The model under review builds one solid part; all positions refer to its coordinate system, in mm. Round coordinates to 2 decimals unless told otherwise and drop trailing zeros. Order: outer loops, then holes, each group sorted by start corner. A loop starts at its lowest first (then second) coordinate and runs counter-clockwise, first axis right, second up. Notation, with made-up numbers: (4, 83) - (35, 83) arc R12 ccw to (35, 91) - close; hole circle Ø11 at (-22, 4). An arc over 180 degrees is marked (long way). One line per question, with ' | ' between items. Start each with the question number.
Item 1: Add section B-B on z = 6. State the section outline as (x, y) points.
Item 2: For L1, parallel to X at y = -23, z = 7.75; L2, parallel to Y at x = -41, z = 1; L3, parallel to Y at x = 123.5, z = 4.75, list the stretches that pass through material, from the lowest coordinate up. Write a range as [from, to].
Item 3: Add section C-C on x = -67.5. State the section outline as (y, z) points.
Item 4: Insertion check: pin 1 Ø3 at (y, z) = (-37, 1.5) entering from -X; pin 2 Ø4 at (y, z) = (25, 4.5) entering from +X; pin 3 Ø3 at (x, z) = (126.5, 4.5) entering from -Y. Each pin has a flat end and moves straight along its axis. Give the tip position at first contact, or say it passes through.
Item 5: Add section A-A on y = 1. State the section outline as (x, z) points.
from build123d import *

# Parameters (mm, degrees)
SKETCH1_W           = 241.3
SKETCH1_H           = 127
BOSS_EXTRUDE1_DEPTH = 10.668
SKETCH3_W           = 91.5
SKETCH3_H           = 91.5
CUT_EXTRUDE1_DEPTH  = 137.757006124
SKETCH4_W           = 19.05
SKETCH4_H           = 15.748
BOSS_EXTRUDE2_DEPTH = 10.668


with BuildPart() as part:
    # Sketch1 → Boss-Extrude1 (new body)
    with BuildSketch(Plane.XY):
        Rectangle(SKETCH1_W, SKETCH1_H)
    extrude(amount=BOSS_EXTRUDE1_DEPTH)

    # Sketch3 → Cut-Extrude1 (cut, through all)
    with BuildSketch(Plane.XY.offset(10.668)):
        with Locations((-53.6875, 0)):
            Rectangle(SKETCH3_W, SKETCH3_H)
        with Locations((53.6875, 0)):
            Rectangle(SKETCH3_W, SKETCH3_H)
    extrude(amount=-CUT_EXTRUDE1_DEPTH, mode=Mode.SUBTRACT)

    # Sketch4 → Boss-Extrude2 (add, through all)
    with BuildSketch(Plane.XY.offset(10.668)):
        with Locations((-130.175, 0)):
            Rectangle(SKETCH4_W, SKETCH4_H)
    boss_extrude2 = extrude(amount=-BOSS_EXTRUDE2_DEPTH)

    # Mirror1: Boss-Extrude2 across plane
    add(boss_extrude2.mirror(Plane(origin=(0, 0, 0), x_dir=(0, 0, 1), z_dir=(1, 0, 0))))


solid = part.part
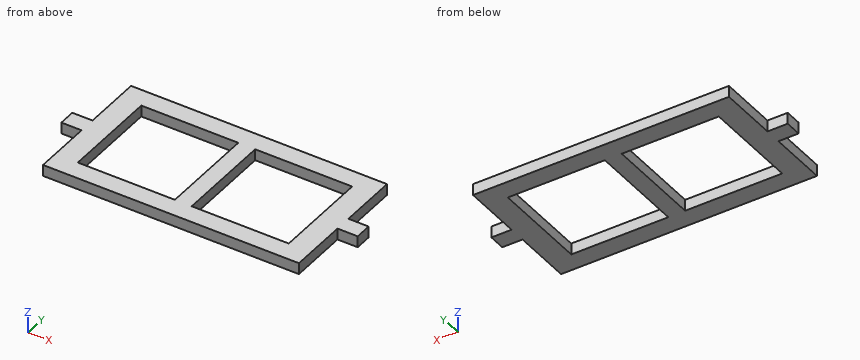
Determined:
1) outline: (-139.7, -7.87) - (-120.65, -7.87) - (-120.65, -63.5) - (120.65, -63.5) - (120.65, -7.87) - (139.7, -7.87) - (139.7, 7.87) - (120.65, 7.87) - (120.65, 63.5) - (-120.65, 63.5) - (-120.65, 7.87) - (-139.7, 7.87) - close; hole (-99.44, -45.75) - (-7.94, -45.75) - (-7.94, 45.75) - (-99.44, 45.75) - close; hole (7.94, -45.75) - (99.44, -45.75) - (99.44, 45.75) - (7.94, 45.75) - close
2) L1: [-120.65, -99.44], [-7.94, 7.94], [99.44, 120.65] | L2: [-63.5, -45.75], [45.75, 63.5] | L3: [-7.87, 7.87]
3) outline: (-63.5, 0) - (-45.75, 0) - (-45.75, 10.67) - (-63.5, 10.67) - close; (45.75, 0) - (63.5, 0) - (63.5, 10.67) - (45.75, 10.67) - close
4) pin 1: x = -120.65 | pin 2: x = 120.65 | pin 3: y = -7.87
5) outline: (-139.7, 0) - (-99.44, 0) - (-99.44, 10.67) - (-139.7, 10.67) - close; (-7.94, 0) - (7.94, 0) - (7.94, 10.67) - (-7.94, 10.67) - close; (99.44, 0) - (139.7, 0) - (139.7, 10.67) - (99.44, 10.67) - close
